```python
from build123d import *

# Parameters (mm, degrees)
F1_DEPTH = 50
F2_DEPTH = 65
F3_R     = 10
F5_ANGLE = -149


with BuildPart() as f1:
    # F0 (on Top) → F1 (new body)
    with BuildSketch(Plane.XY):
        with BuildLine():
            Line((17.6526700227, 31.4716789257), (-36.8578768761, 62.0470002943))
            Line((-36.8578768761, 62.0470002943), (-22.982297547, 38.6886805081))
            ThreePointArc((-22.982297547, 38.6886805081), (-12.9289992244, 38.7823343206), (-7.8751203144, 30.0911959508))
            ThreePointArc((-7.8751203144, 30.0911959508), (-9.1839819445, 25.1450748608), (-12.7679430817, 21.4937113934))
            Line((-12.7679430817, 21.4937113934), (0, 0))
            Line((0, 0), (4.1072919863, -6.9142655162))
            ThreePointArc((4.1072919863, -6.9142655162), (14.160590309, -6.8206117038), (19.214469219, -15.5117500736))
            ThreePointArc((19.214469219, -15.5117500736), (17.9056075888, -20.4578711635), (14.3216464517, -24.1092346309))
            Line((14.3216464517, -24.1092346309), (18.428938438, -31.0235001472))
            Line((18.428938438, -31.0235001472), (45.2960776798, -15.063571295))
            Line((45.2960776798, -15.063571295), (17.6526700227, 31.4716789257))
        make_face()
        with BuildLine():
            Line((-22.982297547, 38.6886805081), (-36.8578768761, 62.0470002943))
            Line((-36.8578768761, 62.0470002943), (-36.0871754027, 0))
            Line((-36.0871754027, 0), (-8.2455254354, -46.8689737481))
            Line((-8.2455254354, -46.8689737481), (18.428938438, -31.0235001472))
            Line((18.428938438, -31.0235001472), (14.3216464517, -24.1092346309))
            ThreePointArc((14.3216464517, -24.1092346309), (0.6169846617, -20.6189273063), (4.1072919863, -6.9142655162))
            Line((4.1072919863, -6.9142655162), (0, 0))
            Line((0, 0), (-12.7679430817, 21.4937113934))
            ThreePointArc((-12.7679430817, 21.4937113934), (-26.4726048717, 24.9840187181), (-22.982297547, 38.6886805081))
        make_face()
    extrude(amount=F1_DEPTH)

    # F0 (on Top) → F2 (join)
    with BuildSketch(Plane.XY):
        with BuildLine():
            ThreePointArc((-7.8751203144, 30.0911959508), (-12.9289992244, 38.7823343206), (-22.982297547, 38.6886805081))
            Line((-22.982297547, 38.6886805081), (-12.7679430817, 21.4937113934))
            ThreePointArc((-12.7679430817, 21.4937113934), (-9.1839819445, 25.1450748608), (-7.8751203144, 30.0911959508))
        make_face()
        with BuildLine():
            Line((-12.7679430817, 21.4937113934), (-22.982297547, 38.6886805081))
            ThreePointArc((-22.982297547, 38.6886805081), (-26.4726048717, 24.9840187181), (-12.7679430817, 21.4937113934))
        make_face()
        with BuildLine():
            Line((14.3216464517, -24.1092346309), (4.1072919863, -6.9142655162))
            ThreePointArc((4.1072919863, -6.9142655162), (0.6169846617, -20.6189273063), (14.3216464517, -24.1092346309))
        make_face()
        with BuildLine():
            ThreePointArc((19.214469219, -15.5117500736), (14.160590309, -6.8206117038), (4.1072919863, -6.9142655162))
            Line((4.1072919863, -6.9142655162), (14.3216464517, -24.1092346309))
            ThreePointArc((14.3216464517, -24.1092346309), (17.9056075888, -20.4578711635), (19.214469219, -15.5117500736))
        make_face()
    extrude(amount=F2_DEPTH)

    # F3
    f3_edges = [f1.edges().sort_by_distance(p)[0] for p in [
        (-27.87512, 30.091196, 65),
        (4.107292, -6.914266, 65),
    ]]
    fillet(f3_edges, radius=F3_R)


with BuildPart() as f1_1:
    # F4: moved
    add(f1.part.moved(Location((-45.5, 15, 0))))


with BuildPart() as f1_2:
    # F5: moved
    add(f1_1.part.rotate(Axis((-0.2039223202, -0.063571295, 25), (0, 0, -1)), F5_ANGLE))


solid = f1_2.part
```
Can you work these out from the model? Positions are in its coordinate system, mm. Coordinates: 2 decimals unless noted, no trailing zeros. Order: outer loops, then holes, each group sorted by start corner. A loop starts at its lowest first (then second) coordinate and runs counter-clockwise, first axis right, second up. Notation, with made-up numbers: (86.25, 64.5) -> (103.25, 64.5) arc R32 cw to (103.25, 90.5) -> close; hole circle Ø2 at (66, 84). An arc over 180 degrees is marked (long way). Write each question's results on one line, items separated by ' | '.
Item 1: I want a section at B-B, the plane z = 17. Write out the boundary of the cut face in (x, y), then the cut area to 3 significant figures.
Results are:
outline: (-0.48, -54.19) -> (30.5, -108.47) -> (61.8, -54.89) -> (62.07, -0.38) -> (-0.2, -0.06) -> close | area: 5,060 mm²
Item 2: I want a section at D-D, the plane y = -16.5. Write out the boundary of the cut face in (x, z).
Results are:
outline: (-0.29, 0) -> (61.99, 0) -> (61.99, 50) -> (40.8, 50) -> (40.8, 55) arc R9.84 ccw to (21.11, 55) -> (21.11, 50) -> (-0.29, 50) -> close
Item 3: I'm going to push flat-ended pins straight in: pin 1 Ø6 at (x, y) = (41.5, -33.5) entering from +Z; pin 2 Ø5 at (x, z) = (28.5, 31.5) entering from +Y; pin 3 Ø4 at (x, y) = (14, -82) entering from -Z; pin 4 Ø1.5 at (y, z) = (-66.5, 42) entering from +X. Where does each tip first touch, or does it pass through?
Results are:
pin 1: z = 50 | pin 2: y = -0.2 | pin 3: z = 0 | pin 4: x = 55.45
Item 4: If we mould it in two halves opening along Y, with no side actions, what happens to faces 1 (the face through (31, -46, 0)), 2 (the face through (31, -46, 50)), 3 (the face through (45.93, -82.06, 24.65))? For each: +Y half, -Y half, draft (parallel to the pull), parting line (faces both ways), or undercut.
Results are:
face 1: draft | face 2: undercut | face 3: -Y half
Item 5: If I drill on line 1 along Z through (x, y) = (30.5, -82); line 2 along Y through (x, z) = (31.5, 60); line 3 along X through (y, z) = (-51, 22), over which ranges is the centre line in solid material (lowest first)?
Results are:
line 1: 0 to 50 | line 2: -79.93 to -62.68, -26.91 to -9.62 | line 3: -0.46 to 61.82
Item 6: I want a section at A-A, the plane y = -70. Write out the boundary of the cut face in (x, z), then the cut area to 3 significant figures.
Results are:
outline: (8.55, 0) -> (52.97, 0) -> (52.97, 50) -> (40.6, 50) -> (40.6, 55) arc R9.91 ccw to (20.77, 55) -> (20.77, 50) -> (8.55, 50) -> close | area: 2,470 mm²
Item 7: I want a section at C-C, the plane x = 28.5. Write out the boundary of the cut face in (y, z).
Results are:
outline: (-104.97, 0) -> (-0.21, 0) -> (-0.21, 50) -> (-8.57, 50) -> (-8.57, 55) arc R9.69 ccw to (-27.96, 55) -> (-27.96, 50) -> (-61.55, 50) -> (-61.55, 55) arc R9.76 ccw to (-81.06, 55) -> (-81.06, 50) -> (-104.97, 50) -> close
